```python
from build123d import *

# Parameters (mm, degrees)
SKETCH1_R           = 6
BOSS_EXTRUDE1_DEPTH = 42
BOSS_EXTRUDE2_START = -24
SKETCH2_R           = 9
BOSS_EXTRUDE2_DEPTH = 2


with BuildPart() as part:
    # Sketch1 → Boss-Extrude1 (new body)
    with BuildSketch(Plane.XY):
        Circle(SKETCH1_R)
    extrude(amount=BOSS_EXTRUDE1_DEPTH)

    # Sketch2 → Boss-Extrude2 (add)
    with BuildSketch(Plane.XY.offset(42).offset(BOSS_EXTRUDE2_START)):
        Circle(SKETCH2_R)
    extrude(amount=BOSS_EXTRUDE2_DEPTH)


solid = part.part
```
Verification items for the finished model (mm, model axes). A direction names the side the tool comes from. Coordinates: 2 decimals unless noted, no trailing zeros. Write each loop counter-clockwise with the first axis right and the second up, starting at its lowest first coordinate (ties: lowest second). Pieces come first, ordered by that corner, then holes. Notation, with made-up numbers: M 18,88 L 57,88 A37 cw 57,126 Z; hole C 37,51 d6. An arc over 180 degrees is marked long. Answer as a JSON object with one key per item and string values. Group by question number.
(1) Cross-section at C-C, the plane z = 19. Record the cut outline in (x, y).
(2) Gauge pin test, flat ends, axial feed: pin 1 (8 mm diameter, centred on x = 5, z = 9.5, fed in from -Y); pin 2 (6 mm diameter, centred on y = -7, z = 23.5, fed in from -X); pin 3 (6 mm diameter, centred on x = -6, y = -1.5, fed in from +Z); pin 4 (1 mm diameter, centred on x = -6, z = 16, fed in from -Y). Record the tip position at first contact, or that the pin passes through.
(3) Material ranges on line 1 (Z direction, x = 6.75, y = -2); line 2 (Y direction, x = 0.25, z = 25.5), recorded low to high.
(4) Tool access check on faces 1 (the face through (0, 0, 0)), 2 (the face through (-6, 0, 9)), 3 (the face through (-6, 0, 31)). Record the directions out of +Z, -Z, +X, -X, +Y, -Y that give a thin tool (end or side, any length) a straight path to the whole face; none if there is none.
(5) Cross-section at A-A, the plane x = 0. Record the cut outline in (y, z), and give its area (3 significant figures).
(6) Cross-section at D-D, the plane z = 3. Record the cut outline in (x, y), and give its area (3 significant figures).
(7) Cross-section at B-B, the plane y = 5. Record the cut outline in (x, z), and give its area (3 significant figures).
Reply:
{
 "1": {"outline": "C 0,0 d18"},
 "2": {"pin 1": "y = -5.92", "pin 2": "x = -4.47", "pin 3": "z = 42", "pin 4": "y = -2.4"},
 "3": {"line 1": "18 to 20", "line 2": "-5.99 to 5.99"},
 "4": {"face 1": "-Z, +X, -X, +Y, -Y", "face 2": "-Z", "face 3": "+Z"},
 "5": {"outline": "M -9,18 L -6,18 L -6,0 L 6,0 L 6,18 L 9,18 L 9,20 L 6,20 L 6,42 L -6,42 L -6,20 L -9,20 Z", "area": "516 mm²"},
 "6": {"outline": "C 0,0 d12", "area": "113 mm²"},
 "7": {"outline": "M -7.48,18 L -3.32,18 L -3.32,0 L 3.32,0 L 3.32,18 L 7.48,18 L 7.48,20 L 3.32,20 L 3.32,42 L -3.32,42 L -3.32,20 L -7.48,20 Z", "area": "295 mm²"}
}
